from build123d import *

# Parameters (mm, degrees)
F0_R     = 80
F1_DEPTH = 101.6
F2_R     = 5.08
F3_R     = 75
F4_DEPTH = 90
F5_R     = 3.175
F6_DEPTH = 127
F7_R     = 3.175
F8_DEPTH = 127


with BuildPart() as f1:
    # F0 (on Front) → F1 (new body)
    with BuildSketch(Plane.XZ):
        Circle(F0_R)
    extrude(amount=-F1_DEPTH)

    # F2
    f2_edges = [f1.edges().sort_by_distance(p)[0] for p in [
        (-80, 0, 0),
    ]]
    fillet(f2_edges, radius=F2_R)

    # F3 (on face) → F4 (cut)
    with BuildSketch(Plane(origin=(0, 101.6, 0), x_dir=(-1, 0, 0), z_dir=(0, 1, 0))):
        Circle(F3_R)
    extrude(amount=-F4_DEPTH, mode=Mode.SUBTRACT)

    # F5 (on Top) → F6 (cut, symmetric)
    with BuildSketch(Plane.XY):
        with Locations((0, 50.8)):
            Circle(F5_R)
    extrude(amount=F6_DEPTH, both=True, mode=Mode.SUBTRACT)

    # F7 (on Right) → F8 (cut, symmetric)
    with BuildSketch(Plane.YZ):
        with Locations((50.8, 0)):
            Circle(F7_R)
    extrude(amount=F8_DEPTH, both=True, mode=Mode.SUBTRACT)


solid = f1.part
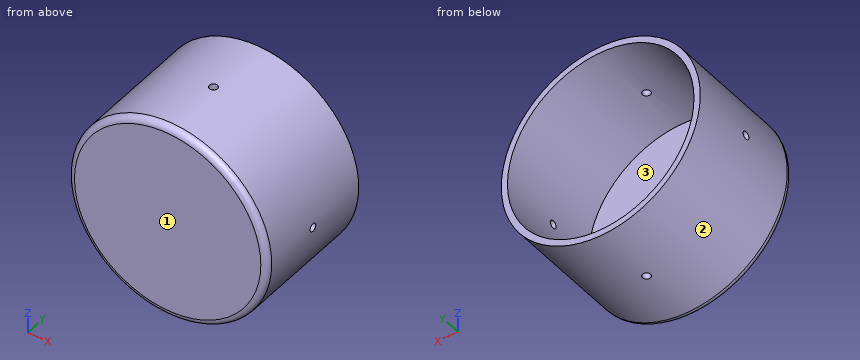
Model file for the job. Use its own axes, mm. Face numbers are marked on the shaded views. Coordinates: 2 decimals unless noted, no trailing zeros. Order: outer loops, then holes, each group sorted by start corner. A loop starts at its lowest first (then second) coordinate and runs counter-clockwise, first axis right, second up. Notation, with made-up numbers: (79.25, 74) -> (104.25, 74) arc R24 cw to (104.25, 113) -> close; hole circle Ø7 at (39, 74.25). An arc over 180 degrees is marked (long way). Return JSON: item names as keys, results as strings. Group by question number.
Item 1: Wall check: line 1 along Z through (x, y) = (1, 76); line 2 along X through (y, z) = (64, 0); line 3 along X through (y, z) = (26, -59.5). Give the ranges that are in metal, low to high. Write a range as [from, to].
Item 2: Flat gauge pins, fed straight in: P1, Ø5, axis at y = 90, z = -17, coming from the -X side; P2, Ø3, axis at x = -39.5, z = -24.5, coming from the -Y side; P3, Ø2, axis at y = 29, z = 5, coming from the -X side; P4, Ø5, axis at y = 21.5, z = -28, coming from the +X side. Where does each tip first touch, or does it go through?
Item 3: Saw through at C-C on y = 18. Write the cut outline in (x, z), then the cut area to 3 significant figures.
Item 4: Saw through at B-B on y = 50.8. Write the cut outline in (x, z) (3 decimals), then the cut area to 3 significant figures.
Item 5: Saw through at A-A on x = 0. Write the cut outline in (y, z) (3 decimals).
Item 6: Pull direction X, two halves, no side cores. Call the marked faces 1, 2 and 3: pulls with the +X half, pulls with the -X half, needs draft (parallel to the pull), parting line crosses it, or undercut.
Values found:
{
 "1": {"line 1": "z = [-79.99, -74.99], [74.99, 79.99]", "line 2": "x = [-80, -75], [75, 80]", "line 3": "x = [-53.48, -45.66], [45.66, 53.48]"},
 "2": {"P1": "stops at x = -78.67", "P2": "stops at y = 0", "P3": "stops at x = -79.9", "P4": "stops at x = 75.83"},
 "3": {"outline": "circle Ø160 at (0, 0); hole circle Ø150 at (0, 0)", "area": "2,430 mm2"},
 "4": {"outline": "(-79.937, -3.175) arc R80 ccw to (-3.175, -79.937) -> (-3.175, -74.933) arc R75 cw to (-74.933, -3.175) -> close; (-79.937, 3.175) -> (-74.933, 3.175) arc R75 cw to (-3.175, 74.933) -> (-3.175, 79.937) arc R80 ccw to start; (3.175, -79.937) arc R80 ccw to (79.937, -3.175) -> (74.933, -3.175) arc R75 cw to (3.175, -74.933) -> close; (3.175, 74.933) arc R75 cw to (74.933, 3.175) -> (79.937, 3.175) arc R80 ccw to (3.175, 79.937) -> close", "area": "2,310 mm2"},
 "5": {"outline": "(0, -74.92) arc R5.08 ccw to (5.08, -80) -> (47.625, -80) -> (47.625, -75) -> (11.6, -75) -> (11.6, 75) -> (47.625, 75) -> (47.625, 80) -> (5.08, 80) arc R5.08 ccw to (0, 74.92) -> close; (53.975, -80) -> (101.6, -80) -> (101.6, -75) -> (53.975, -75) -> close; (53.975, 75) -> (101.6, 75) -> (101.6, 80) -> (53.975, 80) -> close"},
 "6": {"face 1": "needs draft", "face 2": "parting line crosses it", "face 3": "undercut"}
}
